Check sheet for the modelled part. Datum: model origin and axes. Units: mm. A direction names the side the tool comes from. Coordinates: 2 decimals unless noted, no trailing zeros. Write each loop counter-clockwise with the first axis right and the second up, starting at its lowest first coordinate (ties: lowest second). Pieces come first, ordered by that corner, then holes. Notation, with made-up numbers: (-28, -5) - (1, -5) arc R19 cw to (1, 32) - close; hole circle Ø5 at (24, -16). An arc over 180 degrees is marked (long way). Write each question's results on one line, items separated by ' | '.
from build123d import *

# Parameters (mm, degrees)
SKETCH1_R           = 12.5
BOSS_EXTRUDE1_DEPTH = 10
BOSS_EXTRUDE2_DEPTH = 64
SKETCH3_R           = 11
CUT_EXTRUDE1_DEPTH  = 64
BOSS_EXTRUDE3_DEPTH = 10
BOSS_EXTRUDE4_DEPTH = 10


with BuildPart() as part:
    # Sketch1 → Boss-Extrude1 (new body)
    with BuildSketch(Plane.XY):
        with BuildLine():
            Line((-18.634160035, 7.264164081), (-34.222061974, -32.722193067))
            Line((-34.222061974, -32.722193067), (-2.980251959, -44.901203751))
            Line((-2.980251959, -44.901203751), (29.597134129, -36.958099196))
            Line((29.597134129, -36.958099196), (19.430763633, 4.73766025))
            ThreePointArc((19.430763633, 4.73766025), (1.324556426, 19.956090556), (-18.634160035, 7.264164081))
        make_face()
        Circle(SKETCH1_R, mode=Mode.SUBTRACT)
    extrude(amount=BOSS_EXTRUDE1_DEPTH)

    # Sketch2 → Boss-Extrude2 (add)
    with BuildSketch(Plane.XY.offset(10)):
        Polygon((27.228304004, -27.24271738), (29.597134129, -36.958099196), (51.425886213, -31.635755051), (49.057056089, -21.920373235), align=None)
        Polygon((16.450511674, -40.163543501), (29.597134129, -36.958099196), (27.228304004, -27.24271738), (14.081681549, -30.448161684), align=None)
    boss_extrude2 = extrude(amount=BOSS_EXTRUDE2_DEPTH)

    # Sketch3 → Cut-Extrude1 (cut)
    with BuildSketch(Plane(origin=(7.797540371, -31.98037763, 0), x_dir=(0.971538182, 0.236883012, 0), z_dir=(-0.236883012, 0.971538182, 0))):
        with Locations((24.468239022, -32)):
            Circle(SKETCH3_R)
        with BuildLine():
            ThreePointArc((42.468239022, -32), (24.468239022, -50), (6.468239022, -32))
            Line((6.468239022, -32), (6.468239022, -74))
            Line((6.468239022, -74), (42.468239022, -74))
            Line((42.468239022, -74), (42.468239022, -32))
        make_face()
    cut_extrude1 = extrude(amount=-CUT_EXTRUDE1_DEPTH, mode=Mode.SUBTRACT)

    # Mirror1: Boss-Extrude2, Cut-Extrude1 across plane
    add(boss_extrude2.mirror(Plane(origin=(0, 0, 0), x_dir=(0, 0, 1), z_dir=(-0.997804528, 0.066227821, 0))))
    add(cut_extrude1.mirror(Plane(origin=(0, 0, 0), x_dir=(0, 0, 1), z_dir=(-0.997804528, 0.066227821, 0))), mode=Mode.SUBTRACT)

    # Sketch5 → Boss-Extrude3 (add)
    with BuildSketch(Plane(origin=(0, 0, 10), x_dir=(-1, 0, 0), z_dir=(0, 0, -1))):
        Polygon((-49.057056089, -21.920373235), (-51.425886213, -31.635755051), (-29.597134129, -36.958099196), (-27.228304004, -27.24271738), align=None)
    extrude(amount=BOSS_EXTRUDE3_DEPTH)

    # Sketch6 → Boss-Extrude4 (add)
    with BuildSketch(Plane(origin=(0, 0, 10), x_dir=(-1, 0, 0), z_dir=(0, 0, -1))):
        Polygon((30.589979933, -23.405113049), (34.222061974, -32.722193067), (55.155900056, -24.561544323), (51.523818015, -15.244464306), align=None)
    extrude(amount=BOSS_EXTRUDE4_DEPTH)


solid = part.part
1. Sectioned sample at B-B (y = 0). Record the cut outline in (x, z), then the cut area to 3 significant figures.
Values follow:
outline: (-21.47, 0) - (-12.5, 0) - (-12.5, 10) - (-21.47, 10) - close; (12.5, 0) - (20.59, 0) - (20.59, 10) - (12.5, 10) - close | area: 171 mm^2
2. Sectioned sample at C-C (x = 9.5). Record the cut outline in (y, z).
Values follow:
outline: (-41.86, 0) - (-8.12, 0) - (-8.12, 10) - (-41.86, 10) - close; (8.12, 0) - (17.6, 0) - (17.6, 10) - (8.12, 10) - close
3. Sectioned sample at A-A (z = 24.5). Record the cut outline in (x, y), then the cut area to 3 significant figures.
Values follow:
outline: (-55.16, -24.56) - (-45.88, -28.18) - (-42.25, -18.86) - (-51.52, -15.24) - close; (-30.89, -34.02) - (-21.61, -37.64) - (-17.98, -28.32) - (-27.26, -24.7) - close; (14.08, -30.45) - (16.45, -40.16) - (26.12, -37.81) - (23.75, -28.09) - close; (39.39, -24.28) - (41.76, -33.99) - (51.43, -31.64) - (49.06, -21.92) - close | area: 398 mm^2
4. Material ranges on L1, parallel to Z at x = -22, y = -8; L2, parallel to Y at x = -9, z = 3; L3, parallel to Y at x = 0, z = 3, recorded low to high. Write a range as [from, to].
Values follow:
L1: z = [0, 10] | L2: y = [-42.55, -8.67], [8.67, 17.86] | L3: y = [-44.17, -12.5], [12.5, 20]
5. Sectioned sample at D-D (z = 8.5). Record the cut outline in (x, y).
Values follow:
outline: (-55.16, -24.56) - (-2.98, -44.9) - (51.43, -31.64) - (49.06, -21.92) - (27.23, -27.24) - (19.43, 4.74) arc R20 ccw to (-18.63, 7.26) - (-30.59, -23.41) - (-51.52, -15.24) - close; hole circle Ø25 at (0, 0)
6. Draft check along Y on faces 1 (the cylindrical face through (11.923, 3.755, 4.93)), 2 (the flat face through (-24.53, -7.86, 4.93)), 3 (the flat face through (15.25, -35.24, 20.85)). Enter one of: pulls with the +Y half, pulls with the -Y half, needs draft (parallel to the pull), parting line crosses it, or undercut.
Values follow:
face 1: undercut | face 2: pulls with the +Y half | face 3: pulls with the -Y half
7. Go/stop test with flat-tipped pins: pin 1 (5 mm diameter, centred on x = 20, z = 36.5, fed in from +Y); pin 2 (10 mm diameter, centred on x = 1, y = 10, fed in from +Z); pin 3 (10 mm diameter, centred on x = 18, z = 24, fed in from +Y); pin 4 (3 mm diameter, centred on x = 13.5, y = -6.5, fed in from -Z). Record where each tip stops, or that it passes through.
Values follow:
pin 1: stops at y = -28.44 | pin 2: stops at z = 10 | pin 3: stops at y = -28.27 | pin 4: stops at z = 0
8. Access from +Z, -Z, +X, -X, +Y, -Y to the whole of each face (thin tool, end or side, straight path). Record for faces 4 (the flat face through (23.384, -11.476, 4.93)), 5 (the flat face through (-1, -19, 0)), 6 (the flat face through (-19.77, -32.91, 20.85)).
Values follow:
face 4: +Z, -Z, +Y | face 5: -Z, +X, -X, +Y, -Y | face 6: +Z, -Y
